Design review of the part built by this model. Coordinates are the model's own, in mm. Face numbers are marked on the shaded views. A direction names the side the tool comes from. Give positions to 0.01 mm unless a question says otherwise; leave off trailing zeros. Write each loop counter-clockwise with the first axis right and the second up, starting at its lowest first coordinate (ties: lowest second). Pieces come first, ordered by that corner, then holes.
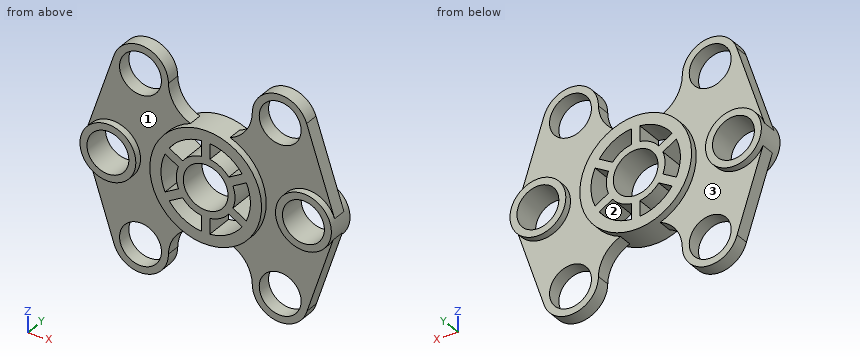
```python
from build123d import *

# Parameters (mm, degrees)
SKETCH1_R             = 40
SKETCH1_R_2           = 16
BOSS_EXTRUDE4_DEPTH   = 10
SKETCH1_R_3           = 20
SKETCH1_R_4           = 15
BOSS_EXTRUDE4_2_DEPTH = 10
BOSS_EXTRUDE4_3_DEPTH = 10
SKETCH1_7_R           = 15
BOSS_EXTRUDE5_DEPTH   = 5


with BuildPart() as part:
    # Sketch1 → Boss-Extrude4 (new, symmetric)
    with BuildSketch(Plane(origin=(0, 0, 0), x_dir=(1, 0, 0), z_dir=(0, 1, 0))):
        with Locations(Location((0, 0, 0), (0, 0, 270))):
            Circle(SKETCH1_R)
        with Locations(Location((0, 0, 0), (0, 0, 270))):
            Circle(SKETCH1_R_2, mode=Mode.SUBTRACT)
        with BuildLine():
            Line((-3, -20.784609691), (-3, -31.859064644))
            ThreePointArc((-3, -31.859064644), (-16, -27.712812921), (-26.090759323, -18.527608533))
            Line((-26.090759323, -18.527608533), (-16.5, -12.990381057))
            ThreePointArc((-16.5, -12.990381057), (-10.5, -18.186533479), (-3, -20.784609691))
        make_face(mode=Mode.SUBTRACT)
        with BuildLine():
            Line((3, -20.784609691), (3, -31.859064644))
            ThreePointArc((3, -31.859064644), (16, -27.712812921), (26.090759323, -18.527608533))
            Line((26.090759323, -18.527608533), (16.5, -12.990381057))
            ThreePointArc((16.5, -12.990381057), (10.5, -18.186533479), (3, -20.784609691))
        make_face(mode=Mode.SUBTRACT)
        with BuildLine():
            Line((-19.5, -7.794228634), (-29.090759323, -13.331456111))
            ThreePointArc((-29.090759323, -13.331456111), (-32, 0), (-29.090759323, 13.331456111))
            Line((-29.090759323, 13.331456111), (-19.5, 7.794228634))
            ThreePointArc((-19.5, 7.794228634), (-21, 0), (-19.5, -7.794228634))
        make_face(mode=Mode.SUBTRACT)
        with BuildLine():
            Line((-16.5, 12.990381057), (-26.090759323, 18.527608533))
            ThreePointArc((-26.090759323, 18.527608533), (-16, 27.712812921), (-3, 31.859064644))
            Line((-3, 31.859064644), (-3, 20.784609691))
            ThreePointArc((-3, 20.784609691), (-10.5, 18.186533479), (-16.5, 12.990381057))
        make_face(mode=Mode.SUBTRACT)
        with BuildLine():
            Line((3, 20.784609691), (3, 31.859064644))
            ThreePointArc((3, 31.859064644), (16, 27.712812921), (26.090759323, 18.527608533))
            Line((26.090759323, 18.527608533), (16.5, 12.990381057))
            ThreePointArc((16.5, 12.990381057), (10.5, 18.186533479), (3, 20.784609691))
        make_face(mode=Mode.SUBTRACT)
        with BuildLine():
            Line((19.5, 7.794228634), (29.090759323, 13.331456111))
            ThreePointArc((29.090759323, 13.331456111), (32, 0), (29.090759323, -13.331456111))
            Line((29.090759323, -13.331456111), (19.5, -7.794228634))
            ThreePointArc((19.5, -7.794228634), (21, 0), (19.5, 7.794228634))
        make_face(mode=Mode.SUBTRACT)
    extrude(amount=BOSS_EXTRUDE4_DEPTH, both=True)



with BuildPart() as body_2:
    # Sketch1 → Boss-Extrude4 2 (new, symmetric)
    with BuildSketch(Plane(origin=(0, 0, 0), x_dir=(1, 0, 0), z_dir=(0, 1, 0))):
        with Locations(Location((70, 0, 0), (0, 0, 270))):
            Circle(SKETCH1_R_3)
        with Locations(Location((70, 0, 0), (0, 0, 270))):
            Circle(SKETCH1_R_4, mode=Mode.SUBTRACT)
    extrude(amount=BOSS_EXTRUDE4_2_DEPTH, both=True)


with BuildPart() as body_3:
    # Sketch1 → Boss-Extrude4 3 (new, symmetric)
    with BuildSketch(Plane(origin=(0, 0, 0), x_dir=(1, 0, 0), z_dir=(0, 1, 0))):
        with Locations(Location((-70, 0, 0), (0, 0, 90))):
            Circle(SKETCH1_R_3)
        with Locations(Location((-70, 0, 0), (0, 0, 270))):
            Circle(SKETCH1_R_4, mode=Mode.SUBTRACT)
    extrude(amount=BOSS_EXTRUDE4_3_DEPTH, both=True)


with BuildPart() as part_1:
    add(part.part)

    add(body_2.part)  # Boss-Extrude5 merges body 2

    add(body_3.part)  # Boss-Extrude5 merges body 3
    # Sketch1_7 → Boss-Extrude5 (add, symmetric)
    # profile 1 of 2: a face of its own
    with BuildSketch(Plane(origin=(0, 0, 0), x_dir=(1, 0, 0), z_dir=(0, 1, 0))):
        with BuildLine():
            ThreePointArc((-14.221544564, -37.38646373), (-40, 0), (-14.221544564, 37.38646373))
            ThreePointArc((-14.221544564, 37.38646373), (-25.532838196, 46.305506483), (-30, 60))
            ThreePointArc((-30, 60), (-47.316842625, 79.819199441), (-69.28006665, 65.317803116))
            Line((-69.28006665, 65.317803116), (-87.870632354, 8.980005528))
            ThreePointArc((-87.870632354, 8.980005528), (-65.385492826, 19.460378299), (-50, 0))
            ThreePointArc((-50, 0), (-66.79635514, -19.741749153), (-88.973665961, -6.32455532))
            Line((-88.973665961, -6.32455532), (-68.973665961, -66.32455532))
            ThreePointArc((-68.973665961, -66.32455532), (-46.79635514, -79.741749153), (-30, -60))
            ThreePointArc((-30, -60), (-25.532838196, -46.305506483), (-14.221544564, -37.38646373))
        make_face()
        with Locations(Location((-50, -60, 0), (0, 0, 270))):
            Circle(SKETCH1_7_R, mode=Mode.SUBTRACT)
        with Locations(Location((-50, 60, 0), (0, 0, 270))):
            Circle(SKETCH1_7_R, mode=Mode.SUBTRACT)
    # profile 2 of 2: a face of its own
    with BuildSketch(Plane(origin=(0, 0, 0), x_dir=(1, 0, 0), z_dir=(0, 1, 0))):
        with BuildLine():
            Line((87.870632354, 8.980005528), (69.28006665, 65.317803116))
            ThreePointArc((69.28006665, 65.317803116), (47.316842625, 79.819199441), (30, 60))
            ThreePointArc((30, 60), (25.532838196, 46.305506483), (14.221544564, 37.38646373))
            ThreePointArc((14.221544564, 37.38646373), (32.930698311, 22.706146937), (40, 0))
            ThreePointArc((40, 0), (32.930698311, -22.706146937), (14.221544564, -37.38646373))
            ThreePointArc((14.221544564, -37.38646373), (25.532838196, -46.305506483), (30, -60))
            ThreePointArc((30, -60), (46.79635514, -79.741749153), (68.973665961, -66.32455532))
            Line((68.973665961, -66.32455532), (88.973665961, -6.32455532))
            ThreePointArc((88.973665961, -6.32455532), (50.051742551, -1.437715109), (87.870632354, 8.980005528))
        make_face()
        with Locations(Location((50, -60, 0), (0, 0, 270))):
            Circle(SKETCH1_7_R, mode=Mode.SUBTRACT)
        with Locations(Location((50, 60, 0), (0, 0, 270))):
            Circle(SKETCH1_7_R, mode=Mode.SUBTRACT)
    extrude(amount=BOSS_EXTRUDE5_DEPTH, both=True)


solid = part_1.part
```
(1) Clearance check with flat-ended pins moving along their axes: P1, Ø1.5, axis at x = 69.5, y = -6.5, coming from the -Z side; P2, Ø9, axis at y = 4.5, z = 28, coming from the -X side; P3, Ø5, axis at x = 20.5, z = -40.5, coming from the -Y side; P4, Ø18, axis at x = 70, z = 0, coming from the +Y side. State where each tip first meets the part, or that it passes through.
Resolved:
P1: stops at z = -20
P2: stops at x = -83.25
P3: stops at y = -5
P4: passes through
(2) Tool access review of the marked faces 1, 2 and 3: name each direction out of +Z, -Z, +X, -X, +Y, -Y from which nothing blocks a thin tool from reaching the whole face with its end or side.
Resolved:
face 1: -Y
face 2: +Y, -Y
face 3: +Y
(3) To check wall thickness, follow L1, parallel to X at y = -0.25, z = 60; L2, parallel to X at y = -0.5, z = -6.5; L3, parallel to X at y = 2, z = 21. State the ranges of each line that lie inside material, in increasing order.
Resolved:
L1: x = -71.08 to -65, -35 to -30, 30 to 35, 65 to 71.08
L2: x = -88.91 to -83.52, -56.48 to -31.33, -19.97 to -14.62, 14.62 to 19.97, 31.33 to 56.48, 83.52 to 88.91
L3: x = -84.08 to -24.15, -3 to 3, 24.15 to 84.08
(4) Consider section A-A, the plane y = -7.25. Give the number of separate pieces and of enclosed holes in the cut face, then the cut area to 3 significant figures.
Resolved:
separate pieces: 3
enclosed holes: 9
area: 3,890 mm2
(5) Consider section C-C, the plane z = 69. Give the boundary of the cut face in (x, y).
Resolved:
outline: (-67.86, -5) - (-62, -5) - (-62, 5) - (-67.86, 5) - close; (-38, -5) - (-32.14, -5) - (-32.14, 5) - (-38, 5) - close; (32.14, -5) - (38, -5) - (38, 5) - (32.14, 5) - close; (62, -5) - (67.86, -5) - (67.86, 5) - (62, 5) - close
(6) Consider section B-B, the plane x = 0. Give the boundary of the cut face in (y, z), then the cut area to 3 significant figures.
Resolved:
outline: (-10, -40) - (10, -40) - (10, -16) - (-10, -16) - close; (-10, 16) - (10, 16) - (10, 40) - (-10, 40) - close
area: 960 mm2
